The figure shows three views and two pictorial views of one solid part (mm, origin at its lowest corner). Answer the questions. Give positions to 0.01 mm unless a question says otherwise; leave off trailing zeros. Write each loop counter-clockwise with the first axis right and the second up, starting at its lowest first coordinate (ties: lowest second). Pieces come first, ordered by that corner, then holes. Notation, with made-up numbers: M 89.25,23 L 134.25,23 A7 cw 134.25,28 Z; hole C 42,50.25 d8. An arc over 180 degrees is marked long. Return JSON: item names as keys, results as strings.
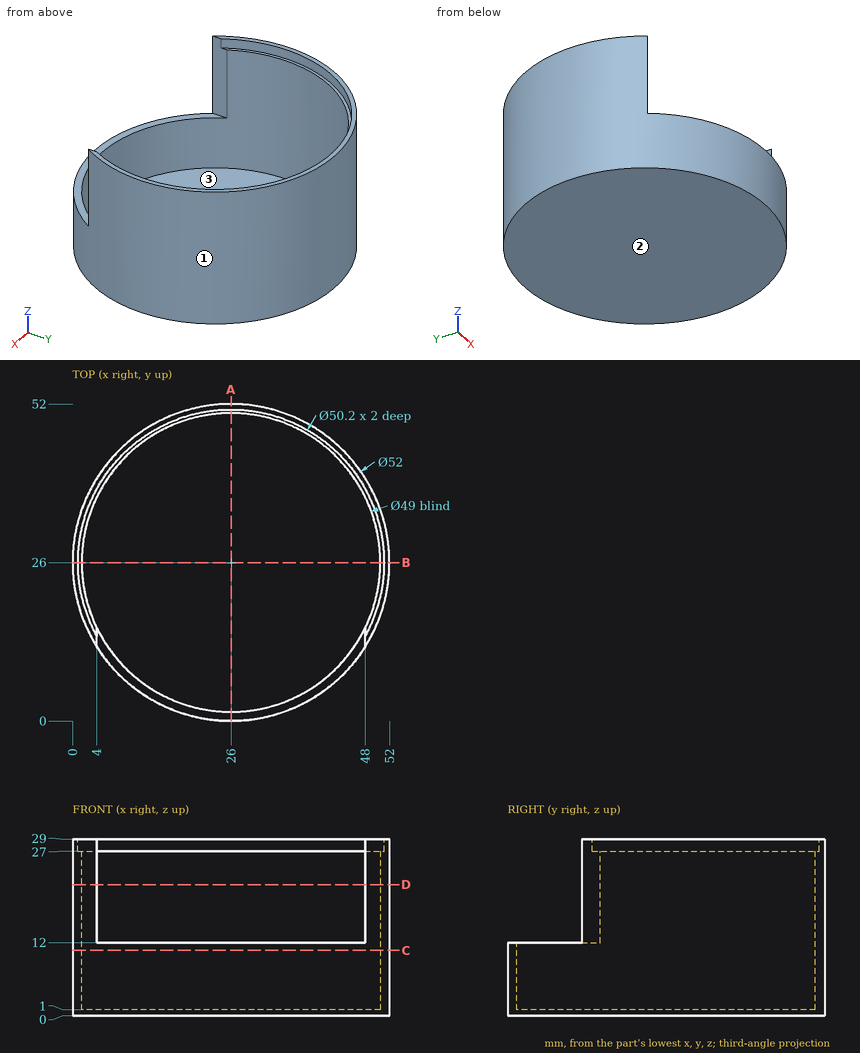
Item 1: A cutting plane is placed at D-D, the plane z = 21.5. Write down the section's boundary in (x, y), plus the area to 3 significant figures.
Geometry results:
{"outline": "M 4,12.14 L 4,15.22 A24.5 cw long 48,15.22 L 48,12.14 A26 ccw long Z", "area": "158 mm2"}
Item 2: A cutting plane is placed at B-B, the plane y = 26. Write down the section's boundary in (x, z), plus the area to 3 significant figures.
Geometry results:
{"outline": "M 0,0 L 52,0 L 52,29 L 51.1,29 L 51.1,27 L 50.5,27 L 50.5,1 L 1.5,1 L 1.5,27 L 0.9,27 L 0.9,29 L 0,29 Z", "area": "134 mm2"}
Item 3: Find the intervals of material crossed by line 1 (Y direction, x = 26, z = 7.25); line 2 (X direction, y = 26, z = 27.5); line 3 (Z direction, x = 30.5, y = 17), in increasing order.
Geometry results:
{"line 1": "y = 0 to 1.5, 50.5 to 52", "line 2": "x = 0 to 0.9, 51.1 to 52", "line 3": "z = 0 to 1"}
Item 4: Given pin 1 Ø5 at (x, z) = (46, 19.5) entering from +Y; pin 2 Ø12 at (x, y) = (22, 7.5) entering from +Z; pin 3 Ø8 at (x, y) = (44, 10.5) entering from -Z; pin 4 Ø3.5 at (y, z) = (13, 23.5) entering from +X, each flat-ended and moving along its own axis, determine where each tip first touches the part or whether it passes through.
Geometry results:
{"pin 1": "stops at y = 45.23", "pin 2": "stops at z = 12", "pin 3": "stops at z = 0", "pin 4": "stops at x = 49.44"}
Item 5: A cutting plane is placed at A-A, the plane x = 26. Write down the section's boundary in (y, z).
Geometry results:
{"outline": "M 0,0 L 52,0 L 52,29 L 51.1,29 L 51.1,27 L 50.5,27 L 50.5,1 L 1.5,1 L 1.5,12 L 0,12 Z"}
Item 6: Determine the mould class of the marked faces 1, 2 and 3 for opening direction Y: +Y half, -Y half, draft (parallel to the pull), parting line (faces both ways), or undercut.
Geometry results:
{"face 1": "parting line", "face 2": "draft", "face 3": "undercut"}
Item 7: A cutting plane is placed at C-C, the plane z = 10.75. Write down the section's boundary in (x, y), plus the area to 3 significant figures.
Geometry results:
{"outline": "C 26,26 d52; hole C 26,26 d49", "area": "238 mm2"}
